Design review of the part shown in the three views and the two pictorial views. Dimensions are in mm from the part's minimum x, y and z. A direction names the side the tool comes from. Give positions to 0.01 mm unless a question says otherwise; leave off trailing zeros. Loops run counter-clockwise (first coordinate to the right, second up) from the corner with the lowest first, then second, coordinate; pieces in that order, holes last.
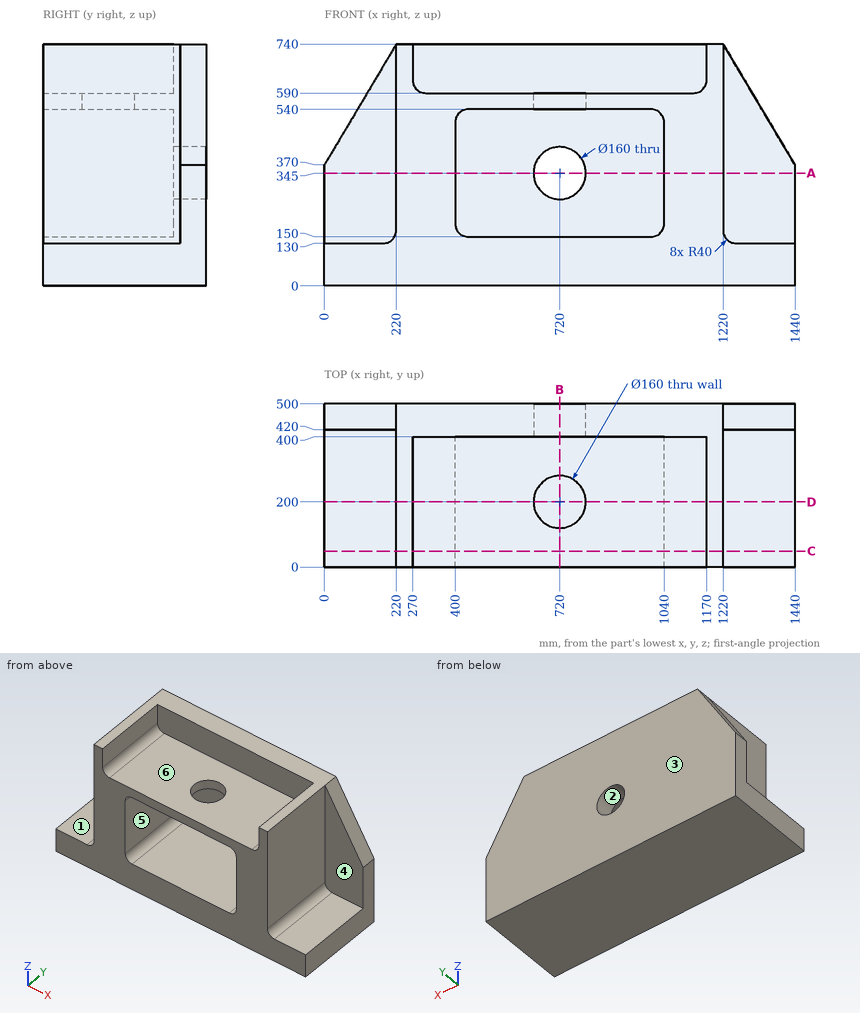
Q1. Insertion check: pin 1 (4 mm diameter, centred on x = 657, z = 156.5, fed in from -Y). The pin has a flat end and moves straight along its axis. Give the tip position at first contact, or say it passes through.
Results:
pin 1: stops at y = 400
Q2. Tool access review of the marked faces 4, 5 and 6: name each direction out of +Z, -Z, +X, -X, +Y, -Y from which nothing blocks a thin tool from reaching the whole face with its end or side.
Results:
face 4: +Z, +X, -Y
face 5: -Y
face 6: +Z, -Y
Q3. Draft analysis for pull direction Z (two halves, no side actions). For the marked faces 1, 2 and 3, state which applies: pulls with the +Z half, pulls with the -Z half, needs draft (parallel to the pull), parting line crosses it, or undercut.
Results:
face 1: pulls with the +Z half
face 2: undercut
face 3: needs draft
Q4. Take a section at D-D (y = 200). Give the boundary of the cut face in (x, z).
Results:
outline: (0, 0) - (1440, 0) - (1440, 130) - (1260, 130) arc R40 cw to (1220, 170) - (1220, 740) - (1170, 740) - (1170, 630) arc R40 cw to (1130, 590) - (800, 590) - (800, 540) - (1000, 540) arc R40 cw to (1040, 500) - (1040, 190) arc R40 cw to (1000, 150) - (440, 150) arc R40 cw to (400, 190) - (400, 500) arc R40 cw to (440, 540) - (640, 540) - (640, 590) - (310, 590) arc R40 cw to (270, 630) - (270, 740) - (220, 740) - (220, 170) arc R40 cw to (180, 130) - (0, 130) - close
Q5. Wall thickness on line 1 (Y direction, x = 720, z = 552.5); line 2 (X direction, y = 34.5, z = 276); line 3 (Y direction, x = 1338, z = 148): over which ranges is each line inside the solid? List them lowest first.
Results:
line 1: y = 0 to 120, 280 to 500
line 2: x = 220 to 400, 1040 to 1220
line 3: y = 420 to 500
Q6. Take a section at C-C (y = 49). Give the boundary of the cut face in (x, z), plus the area to 3 significant figures.
Results:
outline: (0, 0) - (1440, 0) - (1440, 130) - (1260, 130) arc R40 cw to (1220, 170) - (1220, 740) - (1170, 740) - (1170, 630) arc R40 cw to (1130, 590) - (310, 590) arc R40 cw to (270, 630) - (270, 740) - (220, 740) - (220, 170) arc R40 cw to (180, 130) - (0, 130) - close; hole (400, 190) arc R40 ccw to (440, 150) - (1000, 150) arc R40 ccw to (1040, 190) - (1040, 500) arc R40 ccw to (1000, 540) - (440, 540) arc R40 ccw to (400, 500) - close
area: 415,000 mm2
Q7. Take a section at B-B (x = 720). Give the boundary of the cut face in (y, z).
Results:
outline: (0, 0) - (500, 0) - (500, 265) - (400, 265) - (400, 150) - (0, 150) - close; (0, 540) - (120, 540) - (120, 590) - (0, 590) - close; (280, 540) - (400, 540) - (400, 425) - (500, 425) - (500, 740) - (400, 740) - (400, 590) - (280, 590) - close
Q8. Take a section at A-A (z = 345). Give the boundary of the cut face in (x, y).
Results:
outline: (0, 420) - (220, 420) - (220, 0) - (400, 0) - (400, 400) - (640, 400) - (640, 500) - (0, 500) - close; (800, 400) - (1040, 400) - (1040, 0) - (1220, 0) - (1220, 420) - (1440, 420) - (1440, 500) - (800, 500) - close
